Build history of the part. All positions in model axes, mm. A direction names the side the tool comes from. Give positions to 0.01 mm unless a question says otherwise; leave off trailing zeros. Loops run counter-clockwise (first coordinate to the right, second up) from the corner with the lowest first, then second, coordinate; pieces in that order, holes last.
1) Band-saw the part on A-A on y = 0. List the corners of the cut face in (x, z) (3 decimals), then the cut area to 3 significant figures.
2) Two-plate mould, pull along Y, no slides. Class faces 3 (the cylindrical face through (-1.926, -0.607, 5.664)), 4 (the flat face through (2, -5, -4.445)): +Y half, -Y half, draft (parallel to the pull), parting line (faces both ways), or undercut.
3) Band-saw the part on C-C on z = 7. List the corners of the cut face in (x, y), then the cut area to 3 significant figures.
4) Band-saw the part on D-D on z = -0.5. List the corners of the cut face in (x, y).
5) Wall check: line 1 (Y direction, x = 0, z = -1.6); line 2 (Y direction, x = 0, z = 5.1); line 3 (X direction, y = 3.5, z = -1). Give the ranges that are in metal, low to high.
6) Flat gauge pins, fed straight in: P1, Ø5, axis at x = 5, z = -2, coming from the +Y side; P2, Ø4, axis at y = 5, z = 0, coming from the +X side. Where does each tip first touch, or does it go through?
7) 3-axis set-ups, long thin cutter, end or side, ignore diameter. For faces 1 (the cylindrical face through (-4.676, -1.472, -1.483)), 2 (the flat face through (-2, 2, 8.128)): which of +Z, -Z, +X, -X, +Y, -Y reach the whole face in a straight line?
```python
from build123d import *

# Parameters (mm, degrees)
F2_R      = 6.35
F3_DEPTH  = 4.445
F4_R      = 9.525
F5_DEPTH  = 8.128
F6_W      = 38.1
F6_H      = 14.9352
F8_DEPTH  = 25.4
F9_D      = 9.8044
F9_DEPTH  = 5.842
F9_TIP    = 2.9455389266
F10_D     = 4.0386
F11_R     = 22.559553958
F11_R_2   = 6.35
F12_DEPTH = 25.4


with BuildPart() as f3:
    # F2 (on Top) → F3 (new body, through all)
    with BuildSketch(Plane.XY):
        Circle(F2_R)
    extrude(amount=-F3_DEPTH)

    # F4 (on Top) → F5 (join, through all)
    with BuildSketch(Plane.XY):
        Circle(F4_R)
    extrude(amount=F5_DEPTH)

    # F6 (on Top) → F8 (cut)
    with BuildSketch(Plane.XY):
        with Locations((0, -14.9352)):
            Rectangle(F6_W, F6_H)
        with Locations((0, 14.9352)):
            Rectangle(F6_W, F6_H)
    extrude(amount=F8_DEPTH, mode=Mode.SUBTRACT)

    # F9
    with Locations(Plane(origin=(0, 0, -4.445), x_dir=(1, 0, 0), z_dir=(0, 0, -1))):
        with Locations((0, 0)):
            Hole(F9_D / 2, depth=F9_DEPTH)
            with Locations((0, 0, -(F9_DEPTH + F9_TIP / 2))):  # 118° drill point
                Cone(0, F9_D / 2, F9_TIP, mode=Mode.SUBTRACT)

    # F10 (through all)
    with Locations(Plane(origin=(0, 0, -4.445), x_dir=(1, 0, 0), z_dir=(0, 0, -1))):
        with Locations((0, 0)):
            Hole(F10_D / 2)

    # F11 (on offset) → F12 (cut)
    with BuildSketch(Plane.XY.offset(-4.445)):
        Circle(F11_R)
        Circle(F11_R_2, mode=Mode.SUBTRACT)
    extrude(amount=F12_DEPTH, mode=Mode.SUBTRACT)


solid = f3.part
```
Findings below:
1. outline: (-6.35, -4.445) - (-4.902, -4.445) - (-4.902, 1.397) - (-2.019, 3.129) - (-2.019, 8.128) - (-6.35, 8.128) - close; (2.019, 3.129) - (4.902, 1.397) - (4.902, -4.445) - (6.35, -4.445) - (6.35, 8.128) - (2.019, 8.128) - close
1. area: 70.2 mm2
2. face 3: undercut
2. face 4: draft
3. outline: circle Ø12.7 at (0, 0); hole circle Ø4.04 at (0, 0)
3. area: 114 mm2
4. outline: circle Ø12.7 at (0, 0); hole circle Ø9.8 at (0, 0)
5. line 1: y = -6.35 to -4.9, 4.9 to 6.35
5. line 2: y = -6.35 to -2.02, 2.02 to 6.35
5. line 3: x = -5.3 to -3.43, 3.43 to 5.3
6. P1: stops at y = 5.84
6. P2: stops at x = 5.6
7. face 1: -Z
7. face 2: +Z, +X, -X, +Y, -Y
